Verification items for the finished model (mm, model axes). A direction names the side the tool comes from. Give positions to 0.01 mm unless a question says otherwise; leave off trailing zeros. Write each loop counter-clockwise with the first axis right and the second up, starting at its lowest first coordinate (ties: lowest second). Pieces come first, ordered by that corner, then holes. Notation, with made-up numbers: M 3,33 L 16,33 A17 ccw 16,49 Z; hole C 0,5.25 d1. An arc over 180 degrees is marked long. Write item = value, one per line.
Autodesk Inventor part; units mm, degrees
ref_plane "YZ Plane" through (0, 0, 0) normal (1, 0, 0) x (0, 1, 0)
ref_plane "XZ Plane" through (0, 0, 0) normal (0, 1, 0) x (-1, 0, 0)
ref_plane "XY Plane" through (0, 0, 0) normal (0, 0, 1) x (1, 0, 0)
sketch "Sketch1" plane through (0, 0, 0) normal (0, 1, 0) x (-1, 0, 0)
  line L0 (200, 0) -> (-200, 0)
  line L1 (-200, 0) -> (-200, 100)
  line L2 (-200, 100) -> (200, 100)
  line L3 (200, 100) -> (200, 0)
  point P0 (0, 0)
  point P1 (0, 0)
  dimension "Length" = 400
  dimension "Depth" = 100
extrude "Extrusion1" add sketch "Sketch1" along normal mid plane 18
sketch "Sketch2" plane through (200, -9, 100) normal (1, 0, 0) x (0, 0, -1)
  line L0 (0, 0) -> (0, 18)
  line L1 (100, 9) -> (100, 18)
  point P0 (20, 9)
  point P1 (60, 9)
  point P2 (0, 9)
  dimension "d4" = 20
  dimension "d5" = 40
sketch "Sketch3" plane through (0, -9, 0) normal (0, -1, 0) x (1, 0, 0)
  line L0 (200, 0) -> (200, 100)
  line L1 (200, 100) -> (-200, 100)
  line L2 (0, 0) -> (200, 0)
  line L3 (-200, 100) -> (-200, 0)
  point P0 (170, 80)
  point P1 (170, 40)
  point P2 (-170, 60)
  point P3 (-170, 20)
  dimension "HoleDepth" = 30
  dimension "d7" = 20
  dimension "d8" = 40
  dimension "d26" = 20
  dimension "d27" = 40
  dimension "d72" = 30
hole "Hole1" at (200, 0, 80) at (200, 0, 40) direction (-1, 0, 0) diameter 6 depth 30
sketch "Sketch4" plane through (-200, -9, 0) normal (-1, 0, 0) x (0, 0, 1)
  line L0 (100, 18) -> (100, 0)
  line L1 (0, 0) -> (0, 18)
  point P0 (60, 9)
  point P1 (20, 9)
  point P2 (0, 9)
  dimension "d24" = 40
  dimension "d71" = 20
hole "Hole3" at (-200, 0, 60) at (-200, 0, 20) direction (1, 0, 0) diameter 6 depth 30
hole "Hole5" at (170, -9, 80) at (170, -9, 40) direction (0, 1, 0) diameter 15 depth 14
hole "Hole7" at (-170, -9, 60) at (-170, -9, 20) direction (0, 1, 0) diameter 15 depth 14
equation "\"d14\" = HoleDepth"
equation "\"d33\" = HoleDepth"
properties part number "Shelf"
1) Cross-section at B-B on x = -170. Record the boundary of the cut face in (y, z).
From the geometry:
outline = M -9,0 L 9,0 L 9,100 L -9,100 L -9,67.5 L 5,67.5 L 5,52.5 L -9,52.5 L -9,27.5 L 5,27.5 L 5,12.5 L -9,12.5 Z
2) Depth check by flat-ended pin: P1, Ø3.5, axis at y = 0, z = 40, coming from the +X side; P2, Ø13.5, axis at x = -170, z = 60, coming from the -Y side; P3, Ø5, axis at y = 0, z = 80, coming from the +X side. Enter the tip coordinate at first touch or a pass-through.
From the geometry:
P1 = 162.71
P2 = 5
P3 = 162.93
3) Cross-section at A-A on y = 0. Record the boundary of the cut face in (x, z), plus the area to 3 significant figures.
From the geometry:
outline = M -200,0 L 200,0 L 200,37 L 176.87,37 A7.5 cw long 176.87,43 L 200,43 L 200,77 L 176.87,77 A7.5 cw long 176.87,83 L 200,83 L 200,100 L -200,100 L -200,63 L -176.87,63 A7.5 cw long -176.87,57 L -200,57 L -200,23 L -176.87,23 A7.5 cw long -176.87,17 L -200,17 Z
area = 38,700 mm^2
4) Draft check along Z on faces 1 (the flat face through (-170, 5, 20)), 2 (the flat face through (200, 0, 49)), 3 (the flat face through (3, 0, 100)). Enter one of: +Z half, -Z half, draft (parallel to the pull), parting line (faces both ways), or undercut.
From the geometry:
face_1 = undercut
face_2 = draft
face_3 = +Z half
5) Tool access check on faces 4 (the flat face through (-3, 0, 0)), 5 (the cylindrical face through (162.564, -1.902, 80.976)). Record the directions out of +Z, -Z, +X, -X, +Y, -Y that give a thin tool (end or side, any length) a straight path to the whole face; none if there is none.
From the geometry:
face_4 = -Z, +X, -X, +Y, -Y
face_5 = -Y
6) Material ranges on probe 1 along Z at (x, y) = (-170, -4.75); probe 2 along Z at (x, y) = (170, -2); probe 3 along Y at (x, z) = (190, 80), recorded low to high. Write a range as from..to.
From the geometry:
probe_1 = 0..12.5, 27.5..52.5, 67.5..100
probe_2 = 0..32.5, 47.5..72.5, 87.5..100
probe_3 = -9..-3, 3..9
